Part model, mm, in its own coordinate system. Face numbers are marked on the shaded views. Coordinates: 2 decimals unless noted, no trailing zeros. Loops run counter-clockwise (first coordinate to the right, second up) from the corner with the lowest first, then second, coordinate; pieces in that order, holes last. Notation, with made-up numbers: (20.5, 2.5) - (27.5, 2.5) arc R6 ccw to (27.5, 12.5) - close; hole circle Ø5 at (-5, 1.5). An arc over 180 degrees is marked (long way). Use a Markdown table: item, result. Add a question column.
1) Drop flat-ended pins along their axis: P1, Ø1.5, axis at x = 199.5, y = 52, coming from the -Z side; P2, Ø3, axis at x = 527, y = 47.5, coming from the -Z side; P3, Ø1.5, axis at x = 772.5, y = 89, coming from the +Z side. Give the stop position or say it passes through.
2) Pull direction Y, two halves, no side cores. Call the marked faces 1, 2 and 3: +Y half, -Y half, draft (parallel to the pull), parting line (faces both ways), or undercut.
3) Band-saw the part on A-A (x = 711.5). Give the cut face in (y, z).
4) Band-saw the part on C-C (y = 172.5). Give the cut face in (x, z), plus the area to 3 significant figures.
5) Band-saw the part on B-B (z = 0). Give the cut face in (x, y).
6) Band-saw the part on D-D (z = 55.5). Give the cut face in (x, y), plus the area to 3 significant figures.
7) Probe probe 1 along X at (y, z) = (75, 37); probe 2 along Z at (x, y) = (595.5, 145); probe 3 along Z at (x, y) = (1095.5, 93). List the from-to ranges inside material, lowest first. Write a range as [from, to].
from build123d import *

# Parameters (mm, degrees)
SKETCH1_R                = 25
BOSS_EXTRUDE1_DEPTH      = 1200
BOSS_EXTRUDE2_START      = -1198
BOSS_EXTRUDE2_DEPTH      = 1198
BOSS_EXTRUDE3_DEPTH      = 40
BOSS_EXTRUDE3_DEPTH_BACK = 1238
SKETCH3_R                = 25


with BuildPart() as part:
    # Sketch1 → Boss-Extrude1 (new body)
    with BuildSketch(Plane(origin=(0, 0, 0), x_dir=(0, 0, -1), z_dir=(1, 0, 0))):
        Circle(SKETCH1_R)
    extrude(amount=BOSS_EXTRUDE1_DEPTH)

    # Sketch2 → Boss-Extrude2 (add)
    with BuildSketch(Plane(origin=(1200, 0, 0), x_dir=(0, 0, -1), z_dir=(1, 0, 0)).offset(BOSS_EXTRUDE2_START)):
        with BuildLine():
            Line((23.999631554, 7.001263118), (-32.01047339, 198.998315554))
            Line((-32.01047339, 198.998315554), (-14.618110395, 216.390678549))
            Line((-14.618110395, 216.390678549), (-31.616478831, 233.389046986))
            Line((-31.616478831, 233.389046986), (-80.009736499, 184.995789318))
            Line((-80.009736499, 184.995789318), (-23.999631554, -7.001263118))
            ThreePointArc((-23.999631554, -7.001263118), (-7.001263118, 23.999631554), (23.999631554, 7.001263118))
        make_face()
    extrude(amount=BOSS_EXTRUDE2_DEPTH)

    # Sketch3 → Boss-Extrude3 (add, two sides: drawn at the far end of the back side and taken through both)
    with BuildSketch(Plane(origin=(1200, 0, 0), x_dir=(0, 0, -1), z_dir=(1, 0, 0)).offset(-BOSS_EXTRUDE3_DEPTH_BACK)):
        Circle(SKETCH3_R)
    extrude(amount=BOSS_EXTRUDE3_DEPTH + BOSS_EXTRUDE3_DEPTH_BACK)


solid = part.part
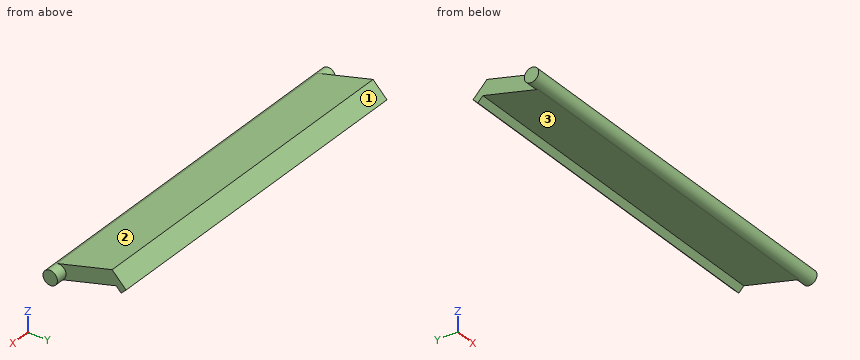
Answer block:
| question | item | result |
|---|---|---|
| 1 | P1 | z = -11.09 |
| 1 | P2 | z = -12.62 |
| 1 | P3 | z = 52.22 |
| 2 | face 1 | +Y half |
| 2 | face 2 | -Y half |
| 2 | face 3 | undercut |
| 3 | outline | (-7, 24) arc R25 ccw to (7, -24) - (199, 32.01) - (216.39, 14.62) - (233.39, 31.62) - (185, 80.01) - close |
| 4 | outline | (2, 24.28) - (1200, 24.28) - (1200, 76.36) - (2, 76.36) - close |
| 4 | area | 62,400 mm2 |
| 5 | outline | (-38, -25) - (1240, -25) - (1240, 25) - (1200, 25) - (1200, 89.27) - (2, 89.27) - (2, 25) - (-38, 25) - close |
| 6 | outline | (2, 100.98) - (1200, 100.98) - (1200, 209.51) - (2, 209.51) - close |
| 6 | area | 130,000 mm2 |
| 7 | probe 1 | [2, 1200] |
| 7 | probe 2 | [16.26, 68.34] |
| 7 | probe 3 | [1.09, 53.17] |
